from build123d import *

# Parameters (mm, degrees)
SKETCH1_R           = 12.7
BOSS_EXTRUDE1_DEPTH = 5
SKETCH2_R           = 6
BOSS_EXTRUDE2_DEPTH = 4.2
SKETCH3_R           = 3
SKETCH3_R_2         = 1.5
CUT_EXTRUDE1_DEPTH  = 14.2
SKETCH5_R           = 1.5
CUT_EXTRUDE2_DEPTH  = 7.1


with BuildPart() as part:
    # Sketch1 → Boss-Extrude1 (new body)
    with BuildSketch(Plane(origin=(0, 0, 0), x_dir=(1, 0, 0), z_dir=(0, 1, 0))):
        with Locations(Location((0, 0, 0), (0, 0, 270))):
            Circle(SKETCH1_R)
    extrude(amount=BOSS_EXTRUDE1_DEPTH)

    # Sketch2 → Boss-Extrude2 (add)
    with BuildSketch(Plane(origin=(0, 5, 0), x_dir=(1, 0, 0), z_dir=(0, 1, 0))):
        with Locations(Location((0, 0, 0), (0, 0, 270))):
            Circle(SKETCH2_R)
    extrude(amount=BOSS_EXTRUDE2_DEPTH)

    # Sketch3 → Cut-Extrude1 (cut)
    with BuildSketch(Plane(origin=(0, 9.2, 0), x_dir=(1, 0, 0), z_dir=(0, 1, 0))):
        with Locations(Location((0, 0, 0), (0, 0, 270))):
            Circle(SKETCH3_R)
        with Locations(Location((-9.5, 0, 0), (0, 0, 270))):
            Circle(SKETCH3_R_2)
        with Locations(Location((-4.75, 8.227241336, 0), (0, 0, 270))):
            Circle(SKETCH3_R_2)
        with Locations(Location((4.75, 8.227241336, 0), (0, 0, 270))):
            Circle(SKETCH3_R_2)
        with Locations(Location((9.5, 0, 0), (0, 0, 270))):
            Circle(SKETCH3_R_2)
        with Locations(Location((4.75, -8.227241336, 0), (0, 0, 270))):
            Circle(SKETCH3_R_2)
        with Locations(Location((-4.75, -8.227241336, 0), (0, 0, 270))):
            Circle(SKETCH3_R_2)
    extrude(amount=-CUT_EXTRUDE1_DEPTH, mode=Mode.SUBTRACT)

    # Sketch5 → Cut-Extrude2 (cut, symmetric)
    with BuildSketch(Plane(origin=(7.125, 0, 4.113620668), x_dir=(0.5000000000000071, 0, -0.8660254037844346), z_dir=(0.8660254037844346, 0, 0.5000000000000071))):
        with Locations((0, 2.5)):
            Circle(SKETCH5_R)
        with Locations((0, 7.2)):
            Circle(SKETCH5_R)
    extrude(amount=CUT_EXTRUDE2_DEPTH, both=True, mode=Mode.SUBTRACT)


solid = part.part
Can you work these out from the model? Positions are in its coordinate system, mm. A direction names the side the tool comes from. Round coordinates to 2 decimals unless told otherwise and drop trailing zeros. Write each loop counter-clockwise with the first axis right and the second up, starting at its lowest first coordinate (ties: lowest second). Pieces come first, ordered by that corner, then holes. Notation, with made-up numbers: (60.5, 77.5) -> (80.5, 77.5) arc R8 ccw to (80.5, 88.5) -> close; hole circle Ø11 at (77, 8). An arc over 180 degrees is marked (long way). Use one line per item in the form item = value. Start each with the question number.
Q1. We'd pull the mould along Z, two halves only. Please class faces 3 (the face through (-5.857, 7.071, -1.301)), 4 (the face through (-3, 0, 3)), 5 (the face through (8, 3, 0)): +Z half, -Z half, draft (parallel to the pull), parting line (faces both ways), or undercut.
Q2. If I drill on probe 1 along X at (y, z) = (3.35, 0); probe 2 along X at (y, z) = (2.25, -7.75); probe 3 along X at (y, z) = (2, 0.5), over which ranges is the centre line in solid material (lowest first)? Write a range as [from, to].
Q3. Imagine slicing it at D-D (x = -4.75). Please give me the cut outline in (y, z), then the cut area to 3 significant figures.
Q4. Which directions (+Z, -Z, +X, -X, +Y, -Y) give clear straight access to the entire face, cutting with the end or side of a thin tool? Please do faces 1 (the face through (3, 5, 5.5)), 2 (the face through (-2.93, 4.66, -0.65)).
Q5. Imagine slicing it at A-A (x = 0). Please give me the cut outline in (y, z), then the cut area to 3 significant figures.
Q6. Imagine slicing it at C-C (y = 2). Please give me the cut outline in (x, z).
Q7. Imagine slicing it at B-B (z = -2.25). Please give me the cut outline in (x, y).
Q8. I'm going to push flat-ended pins straight in: P1, Ø2.5, axis at x = -4.75, z = -8.23, coming from the +Y side; P2, Ø4, axis at x = 4.75, z = 8.23, coming from the +Y side; P3, Ø2, axis at x = -8, y = 3, coming from the +Z side; P4, Ø2, axis at x = 9.5, y = 5, coming from the -Z side. Where does each tip first touch, or does it pass through?
Worked out:
q1.face_3 = parting line
q1.face_4 = draft
q1.face_5 = undercut
q2.probe_1 = [-12.7, -11], [-8, -3], [3, 8], [11, 12.7]
q2.probe_2 = [-10.06, -6.17], [-3.33, 3.33], [6.17, 10.06]
q2.probe_3 = [-12.69, -10.91], [-8.09, -2.96], [3.69, 8.09], [10.91, 12.69]
q3.outline = (0, -11.78) -> (5, -11.78) -> (5, -9.73) -> (0, -9.73) -> close; (0, -6.73) -> (5, -6.73) -> (5, -3.67) -> (9.2, -3.67) -> (9.2, 3.67) -> (5, 3.67) -> (5, 6.73) -> (0, 6.73) -> close; (0, 9.73) -> (5, 9.73) -> (5, 11.78) -> (0, 11.78) -> close
q3.area = 119 mm^2
q4.face_1 = +Y
q4.face_2 = +Y, -Y
q5.outline = (0, -12.7) -> (5, -12.7) -> (5, -6) -> (9.2, -6) -> (9.2, -3) -> (0, -3) -> close; (0, 3) -> (9.2, 3) -> (9.2, 6) -> (5, 6) -> (5, 12.7) -> (0, 12.7) -> close
q5.area = 122 mm^2
q6.outline = (1.58, 2.55) -> (10.22, 7.54) arc R12.7 ccw (long way) to (11.64, 5.09) -> (3, 0.1) arc R3 cw (long way) to start; hole circle Ø3 at (-9.5, 0); hole circle Ø3 at (-4.75, -8.23); hole circle Ø3 at (-4.75, 8.23); hole circle Ø3 at (4.75, -8.23); hole circle Ø3 at (4.75, 8.23); hole circle Ø3 at (9.5, 0)
q7.outline = (-12.5, 0) -> (-1.98, 0) -> (-1.98, 9.2) -> (-5.56, 9.2) -> (-5.56, 5) -> (-12.5, 5) -> close; (1.98, 0) -> (12.5, 0) -> (12.5, 5) -> (5.56, 5) -> (5.56, 9.2) -> (1.98, 9.2) -> close
q8.P1 = through
q8.P2 = 5
q8.P3 = 10.6
q8.P4 = -9.44
